Geometry check sheet. Reference: the model listing, model coordinates, mm. A direction names the side the tool comes from. Give positions to 0.01 mm unless a question says otherwise; leave off trailing zeros. Loops run counter-clockwise (first coordinate to the right, second up) from the corner with the lowest first, then second, coordinate; pieces in that order, holes last. Notation, with made-up numbers: (47.25, 12) -> (78.25, 12) arc R9 ccw to (78.25, 25) -> close; hole circle Ø3 at (87.25, 59.5). An arc over 180 degrees is marked (long way). One line per item, written item: value. Start each with the question number.
(1) Gauge pin test, flat ends, axial feed: pin 1 Ø1.2 at (x, y) = (3.5, -1) entering from +Z; pin 2 Ø1.2 at (x, z) = (3, 12.5) entering from +Y; pin 3 Ø1.5 at (y, z) = (36.5, 10) entering from +X; pin 4 Ø3 at (y, z) = (-31.5, 11.5) entering from -X. Record the tip position at first contact, or that the pin passes through.
(2) Scan lines: line 1 along X through (y, z) = (-11.5, 8.25); line 2 along X through (y, z) = (3, 3); line 3 along Z through (x, y) = (-3, -20.5). Record each from-to range of solid material in increasing order. Write a range as from..to.
(3) Sectioned sample at C-C, the plane z = 11.5. State how many separate pieces and enclosed holes the cut face has, then the cut area to 3 significant figures.
(4) Tool access check on faces 1 (the face through (3, 25, 12)), 2 (the face through (-16.64, 43.4, 1.48)), 3 (the face through (10, -42.5, 1)). Record the directions out of +Z, -Z, +X, -X, +Y, -Y that give a thin tool (end or side, any length) a straight path to the whole face; none if there is none.
(5) Draft check along Z on faces 4 (the face through (10, 42.5, 1)), 5 (the face through (-2.896, -42.719, 12.294)), 6 (the face through (-2.896, 33.408, 12.101)). Enter one of: pulls with the +Z half, pulls with the -Z half, needs draft (parallel to the pull), parting line crosses it, or undercut.
(6) Sectioned sample at A-A, the plane x = -10. Record the cut outline in (y, z), then the cut area to 3 significant figures.
(7) Sectioned sample at D-D, the plane y = 24. Record the cut outline in (x, z), then the cut area to 4 significant figures.
(8) Sectioned sample at B-B, the plane y = -50. Record the cut outline in (x, z).
from build123d import *

# Parameters (mm, degrees)
SKETCH_R     = 2
PAD_DEPTH    = 3
SKETCH001_W  = 4.15
SKETCH001_H  = 90
PAD001_DEPTH = 11.7
SKETCH002_R  = 2
SKETCH002_W  = 50
SKETCH002_H  = 6
POCKET_DEPTH = 15
SKETCH003_W  = 4.09
SKETCH003_H  = 90
PAD002_DEPTH = 3.5
FILLET_R     = 8


with BuildPart() as part:
    # Sketch → Pad (new body)
    with BuildSketch(Plane.XY):
        with BuildLine():
            Line((-14.5, 57.5), (14.5, 57.5))
            ThreePointArc((17.5, 54.5), (16.62132, 56.62132), (14.5, 57.5))
            Line((17.5, 54.5), (17.5, 45.5))
            ThreePointArc((14.5, 42.5), (16.62132, 43.37868), (17.5, 45.5))
            Line((14.5, 42.5), (5, 42.5))
            Line((5, 42.5), (5, -42.5))
            Line((5, -42.5), (14.5, -42.5))
            ThreePointArc((17.5, -45.5), (16.62132, -43.37868), (14.5, -42.5))
            Line((17.5, -45.5), (17.5, -54.5))
            ThreePointArc((14.5, -57.5), (16.62132, -56.62132), (17.5, -54.5))
            Line((14.5, -57.5), (-14.5, -57.5))
            ThreePointArc((-17.5, -54.5), (-16.62132, -56.62132), (-14.5, -57.5))
            Line((-17.5, -54.5), (-17.5, -45.5))
            ThreePointArc((-14.5, -42.5), (-16.62132, -43.37868), (-17.5, -45.5))
            Line((-5, -42.5), (-14.5, -42.5))
            Line((-5, 42.5), (-5, -42.5))
            Line((-14.5, 42.5), (-5, 42.5))
            ThreePointArc((-17.5, 45.5), (-16.62132, 43.37868), (-14.5, 42.5))
            Line((-17.5, 45.5), (-17.5, 54.5))
            ThreePointArc((-14.5, 57.5), (-16.62132, 56.62132), (-17.5, 54.5))
        make_face()
        with Locations((-10, 50)):
            Circle(SKETCH_R, mode=Mode.SUBTRACT)
        with Locations((10, 50)):
            Circle(SKETCH_R, mode=Mode.SUBTRACT)
        with Locations((-10, -50)):
            Circle(SKETCH_R, mode=Mode.SUBTRACT)
        with Locations((10, -50)):
            Circle(SKETCH_R, mode=Mode.SUBTRACT)
    extrude(amount=PAD_DEPTH)

    # Sketch001 → Pad001 (join)
    with BuildSketch(Plane.XY.offset(3)):
        with Locations((-2.925, 0)):
            Rectangle(SKETCH001_W, SKETCH001_H)
        with Locations((2.925, 0)):
            Rectangle(SKETCH001_W, SKETCH001_H)
    extrude(amount=PAD001_DEPTH)

    # Sketch002 → Pocket (cut)
    with BuildSketch(Plane.YZ.offset(5)):
        with Locations((-31.5, 11.5)):
            Circle(SKETCH002_R)
        with Locations((31.5, 11.5)):
            Circle(SKETCH002_R)
        with Locations((0, 12)):
            Rectangle(SKETCH002_W, SKETCH002_H)
    extrude(amount=-POCKET_DEPTH, mode=Mode.SUBTRACT)

    # Sketch003 → Pad002 (join)
    with BuildSketch(Plane.XY.offset(3)):
        with Locations((0.341939, 0)):
            Rectangle(SKETCH003_W, SKETCH003_H)
    extrude(amount=PAD002_DEPTH)

    # Fillet
    fillet_edges = [part.edges().sort_by_distance(p)[0] for p in [
        (-2.925, -45, 14.7),
        (2.925, -45, 14.7),
        (2.925, 45, 14.7),
        (-2.925, 45, 14.7),
    ]]
    fillet(fillet_edges, radius=FILLET_R)


solid = part.part
Calculated:
1. pin 1: stops at z = 9
1. pin 2: stops at y = 43.08
1. pin 3: stops at x = 5
1. pin 4: passes through
2. line 1: x = -5..-0.85, 0.85..5
2. line 2: x = -5..5
2. line 3: z = 0..9
3. separate pieces: 8
3. enclosed holes: 0
3. area: 239 mm2
4. face 1: +Z, +X, -X
4. face 2: +Z, -Z, -X
4. face 3: +Z, -Z, +X
5. face 4: needs draft
5. face 5: pulls with the +Z half
5. face 6: undercut
6. outline: (-57.5, 0) -> (-52, 0) -> (-52, 3) -> (-57.5, 3) -> close; (-48, 0) -> (-42.5, 0) -> (-42.5, 3) -> (-48, 3) -> close; (42.5, 0) -> (48, 0) -> (48, 3) -> (42.5, 3) -> close; (52, 0) -> (57.5, 0) -> (57.5, 3) -> (52, 3) -> close
6. area: 66.0 mm2
7. outline: (-5, 0) -> (5, 0) -> (5, 9) -> (0.85, 9) -> (0.85, 6.5) -> (-0.85, 6.5) -> (-0.85, 9) -> (-5, 9) -> close
7. area: 85.75 mm2
8. outline: (-17.5, 0) -> (-12, 0) -> (-12, 3) -> (-17.5, 3) -> close; (-8, 0) -> (8, 0) -> (8, 3) -> (-8, 3) -> close; (12, 0) -> (17.5, 0) -> (17.5, 3) -> (12, 3) -> close
